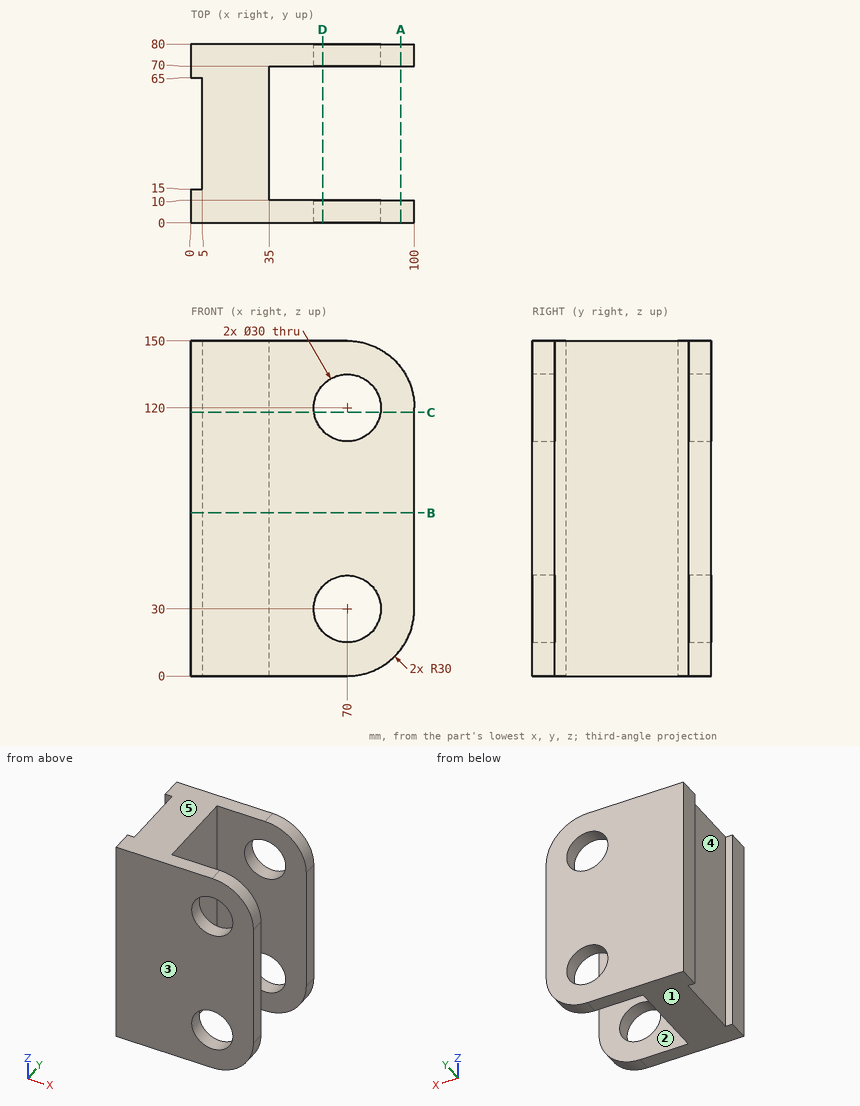
Source: three-view drawing plus pictorial views. Frame: mm from the lowest corner of the part. A direction names the side the tool comes from. Coordinates: 2 decimals unless noted, no trailing zeros. Loops run counter-clockwise (first coordinate to the right, second up) from the corner with the lowest first, then second, coordinate; pieces in that order, holes last. Notation, with made-up numbers: (-8, -17.5) - (38, -17.5) arc R23 ccw to (38, 8.5) - close; hole circle Ø2 at (-7.75, 76). An arc over 180 degrees is marked (long way). One line per item, written item: value. Start each with the question number.
1. Section D-D (x = 59). Return the cut outline in (y, z), and give its area (3 significant figures).
2. Section B-B (z = 73). Return the cut outline in (x, y), and give its area (3 significant figures).
3. Section C-C (z = 118). Return the cut outline in (x, y).
4. Mould query, pull axis Y, two halves, no side actions, for the marked faces 3, 4 and 5. Classes: pulls with the +Y half, pulls with the -Y half, needs draft (parallel to the pull), parting line crosses it, or undercut.
5. Section A-A (x = 94). Return the cut outline in (y, z), and give its area (3 significant figures).
6. Set-up query: the marked faces 1 and 2. Return all of +Z, -Z, +X, -X, +Y, -Y with unobstructed straight access to the full face (end or side cutting, diameter ignored); none if empty.
7. Contact query for flat-ended pins moving along their axis: P1, Ø3, axis at y = 12, z = 79, coming from the +X side; P2, Ø5, axis at x = 51, z = 78, coming from the -Y side; P3, Ø4, axis at y = 24.5, z = 48, coming from the -X side; P4, Ø8, axis at x = 77.5, y = 68, coming from the +Z side. Output: stop coordinate, or through.
8. Ray query, L1, parallel to X at y = 7.5, z = 120; L2, parallel to Y at x = 42, z = 48; L3, parallel to Z at x = 62.5, y = 71.5. Return the intervals inside material, ascending.
Verdict:
1. outline: (0, 0) - (10, 0) - (10, 19.8) - (0, 19.8) - close; (0, 40.2) - (10, 40.2) - (10, 109.8) - (0, 109.8) - close; (0, 130.2) - (10, 130.2) - (10, 150) - (0, 150) - close; (70, 0) - (80, 0) - (80, 19.8) - (70, 19.8) - close; (70, 40.2) - (80, 40.2) - (80, 109.8) - (70, 109.8) - close; (70, 130.2) - (80, 130.2) - (80, 150) - (70, 150) - close
1. area: 2,180 mm2
2. outline: (0, 0) - (100, 0) - (100, 10) - (35, 10) - (35, 70) - (100, 70) - (100, 80) - (0, 80) - (0, 65) - (5, 65) - (5, 15) - (0, 15) - close
2. area: 3,850 mm2
3. outline: (0, 0) - (55.13, 0) - (55.13, 10) - (35, 10) - (35, 70) - (55.13, 70) - (55.13, 80) - (0, 80) - (0, 65) - (5, 65) - (5, 15) - (0, 15) - close; (84.87, 0) - (100, 0) - (100, 10) - (84.87, 10) - close; (84.87, 70) - (100, 70) - (100, 80) - (84.87, 80) - close
4. face 3: pulls with the -Y half
4. face 4: undercut
4. face 5: needs draft
5. outline: (0, 12) - (10, 12) - (10, 138) - (0, 138) - close; (70, 12) - (80, 12) - (80, 138) - (70, 138) - close
5. area: 2,520 mm2
6. face 1: -Z, +X, -X, +Y, -Y
6. face 2: +Z, -Z, +X
7. P1: stops at x = 35
7. P2: stops at y = 0
7. P3: stops at x = 5
7. P4: stops at z = 149.73
8. L1: x = 0 to 55, 85 to 100
8. L2: y = 0 to 10, 70 to 80
8. L3: z = 0 to 17.01, 42.99 to 107.01, 132.99 to 150
